Check sheet for the drawn part. Datum: minimum x, y, z corner. Units: mm. A direction names the side the tool comes from. Coordinates: 2 decimals unless noted, no trailing zeros. Loops run counter-clockwise (first coordinate to the right, second up) from the corner with the lowest first, then second, coordinate; pieces in that order, holes last. Notation, with made-up numbers: M 4,-32.75 L 45,-32.75 A17 cw 45,-6.75 Z; hole C -33,28 d2. An arc over 180 degrees is marked long. Use CSV: the item, a comma, the result in double quotes. Start each with the question number.
(1) Set-up check for the marked faces 1, 2 and 3: record each of +Z, -Z, +X, -X, +Y, -Y from which the full face is reachable in a straight line by a thin tool's end or side.
(2) Section check C-C on y = 20.5. Record the cut outline in (x, z).
(3) Go/stop test with flat-tipped pins: pin 1 Ø3 at (y, z) = (169, 19.5) entering from -X; pin 2 Ø5 at (x, y) = (198.5, 160.5) entering from -Z; pin 3 Ø6 at (y, z) = (48, 15) entering from -X (1 decimal); pin 4 Ø12.5 at (y, z) = (20, 6.5) entering from -X. Record where each tip stops, or that it passes through.
(4) Draft check along X on the marked faces 4, 5 and 6. Enter one of: pulls with the +X half, pulls with the -X half, needs draft (parallel to the pull), parting line crosses it, or undercut.
(5) Section check A-A on z = 3. Record the cut outline in (x, y) (1 decimal).
(6) Section check B-B on x = 204. Record the cut outline in (y, z), and give its area (3 significant figures).
(7) Scan lines: line 1 (X direction, y = 132.5, z = 17) (1 decimal); line 2 (X direction, y = 135.5, z = 19.25); line 3 (Z direction, x = 167.5, y = 172.5). Record each from-to range of solid material in increasing order.
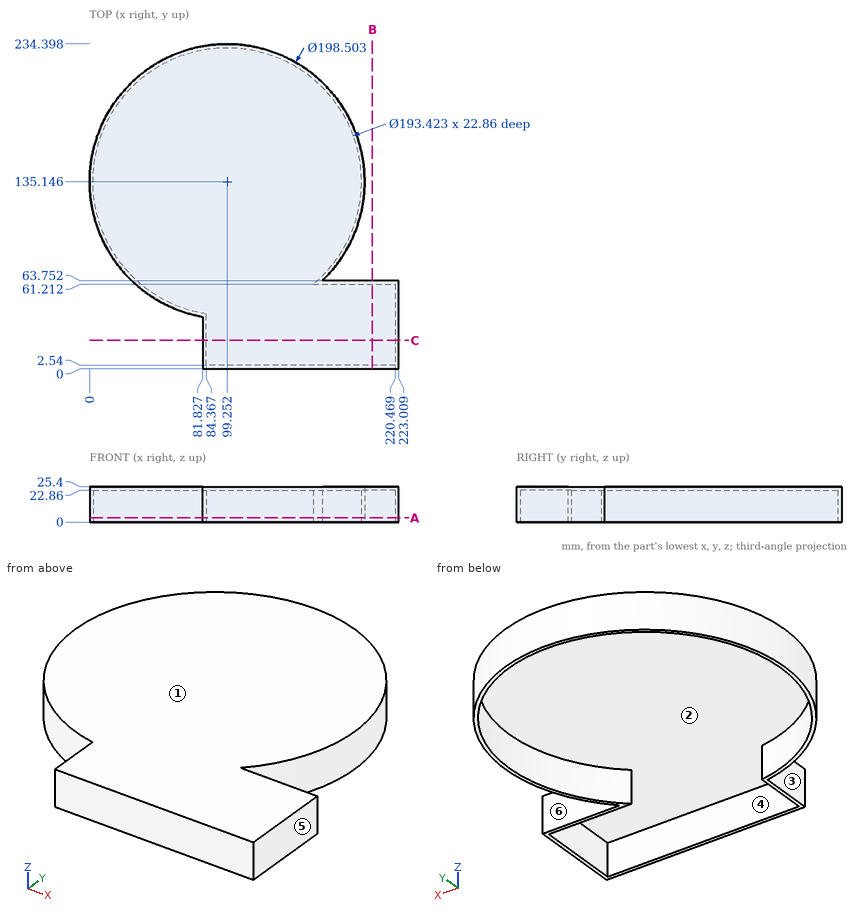
Outcome:
1,face 1,"+Z, +X, -X, +Y, -Y"
1,face 2,"-Z"
1,face 3,"+Z, -Z, -X, -Y"
2,outline,"M 81.83,0 L 84.37,0 L 84.37,22.86 L 220.47,22.86 L 220.47,0 L 223.01,0 L 223.01,25.4 L 81.83,25.4 Z"
3,pin 1,"stops at x = 5.42"
3,pin 2,"passes through"
3,pin 3,"stops at x = 46.6"
3,pin 4,"stops at x = 81.83"
4,face 4,"undercut"
4,face 5,"pulls with the +X half"
4,face 6,"needs draft"
5,outline,"M 81.8,0 L 223,0 L 223,63.8 L 168.2,63.8 A99.3 ccw long 81.8,37.4 Z; hole M 84.4,2.5 L 220.5,2.5 L 220.5,61.2 L 161.6,61.2 A96.7 ccw long 84.4,39.6 Z"
6,outline,"M 0,0 L 2.54,0 L 2.54,22.86 L 61.21,22.86 L 61.21,0 L 63.75,0 L 63.75,25.4 L 0,25.4 Z"
6,area,"278 mm²"
7,line 1,"x = 0 to 2.6, 195.9 to 198.5"
7,line 2,"x = 0 to 2.54, 195.96 to 198.5"
7,line 3,"z = 22.86 to 25.4"
